```python
from build123d import *

# Parameters (mm, degrees)
SKETCH2_R           = 1.5
BOSS_EXTRUDE3_DEPTH = 3
BOSS_EXTRUDE4_DEPTH = 3
SKETCH4_R           = 1.25
CUT_EXTRUDE1_DEPTH  = 3
BOSS_EXTRUDE5_DEPTH = 3
CUT_EXTRUDE2_DEPTH  = 3
BOSS_EXTRUDE6_START = -3
SKETCH7_R           = 1.5
SKETCH7_R_2         = 1.25
BOSS_EXTRUDE6_DEPTH = 3
CUT_EXTRUDE3_DEPTH  = 10
BOSS_EXTRUDE7_DEPTH = 3


with BuildPart() as part:
    # Sketch2 → Boss-Extrude3 (new body)
    with BuildSketch(Plane.XY):
        with BuildLine():
            Line((-69.686145903, 39.746340023), (-34.686145903, 39.746340023))
            Line((-34.686145903, 39.746340023), (-34.686145903, 59.746340023))
            Line((-34.686145903, 59.746340023), (-69.686145903, 49.746340023))
            ThreePointArc((-69.686145903, 49.746340023), (-74.686145903, 44.746340023), (-69.686145903, 39.746340023))
        make_face()
        with Locations((-69.686145903, 44.746340023)):
            Circle(SKETCH2_R, mode=Mode.SUBTRACT)
    extrude(amount=BOSS_EXTRUDE3_DEPTH)

    # Sketch3 → Boss-Extrude4 (add)
    with BuildSketch(Plane.XY.offset(3)):
        with BuildLine():
            Line((-64.686145903, 39.746340023), (-59.686145903, 39.746340023))
            Line((-59.686145903, 39.746340023), (-54.686145903, 39.746340023))
            ThreePointArc((-54.686145903, 39.746340023), (-59.686145903, 34.746340023), (-64.686145903, 39.746340023))
        make_face()
    extrude(amount=-BOSS_EXTRUDE4_DEPTH)

    # Sketch4 → Cut-Extrude1 (cut)
    with BuildSketch(Plane.XY.offset(3)):
        with Locations((-59.686145903, 39.746340023)):
            Circle(SKETCH4_R)
    extrude(amount=-CUT_EXTRUDE1_DEPTH, mode=Mode.SUBTRACT)

    # Sketch5 → Boss-Extrude5 (add)
    with BuildSketch(Plane.XY.offset(3)):
        Polygon((-34.686145903, 59.746340023), (-34.686145903, 62.746340023), (-69.686145903, 49.746340023), align=None)
    extrude(amount=-BOSS_EXTRUDE5_DEPTH)

    # Sketch6 → Cut-Extrude2 (cut)
    with BuildSketch(Plane.XY.offset(3)):
        Polygon((-34.686145903, 39.746340023), (-35.686145903, 39.746340023), (-35.686145903, 63.560014977), (-33.928047703, 63.560014977), (-33.928047703, 39.746340023), align=None)
    extrude(amount=-CUT_EXTRUDE2_DEPTH, mode=Mode.SUBTRACT)

    # Sketch7 → Boss-Extrude6 (add)
    with BuildSketch(Plane.XY.offset(3).offset(BOSS_EXTRUDE6_START)):
        with Locations((-69.686145903, 44.746340023)):
            Circle(SKETCH7_R)
        with Locations((-69.686145903, 44.746340023)):
            Circle(SKETCH7_R_2, mode=Mode.SUBTRACT)
    extrude(amount=BOSS_EXTRUDE6_DEPTH)

    # Sketch8 → Cut-Extrude3 (cut)
    with BuildSketch(Plane.XY.offset(3)):
        Polygon((-69.686145903, 49.746340023), (-45.686145903, 49.746340023), (-45.686145903, 58.660625737), align=None)
    extrude(amount=-CUT_EXTRUDE3_DEPTH, mode=Mode.SUBTRACT)

    # Sketch9 → Boss-Extrude7 (add)
    with BuildSketch(Plane.XY.offset(3)):
        with BuildLine():
            Line((-59.686145903, 34.746340023), (-54.686145903, 34.746340023))
            Line((-54.686145903, 34.746340023), (-54.686145903, 39.746340023))
            ThreePointArc((-54.686145903, 39.746340023), (-56.150611997, 36.210806117), (-59.686145903, 34.746340023))
        make_face()
    extrude(amount=-BOSS_EXTRUDE7_DEPTH)


solid = part.part
```
Build history of the part. All positions in model axes, mm. A direction names the side the tool comes from. Round coordinates to 2 decimals unless told otherwise and drop trailing zeros. Write each loop counter-clockwise with the first axis right and the second up, starting at its lowest first coordinate (ties: lowest second). Pieces come first, ordered by that corner, then holes.
1) Drill centre lines: probe 1 along X at (y, z) = (53.5, 2.25); probe 2 along Y at (x, z) = (-48.5, 0.45); probe 3 along Y at (x, z) = (-55, 0.6). Where is each one in solid material? Low to high.
2) Band-saw the part on B-B, the plane y = 45.25. List the corners of the cut face in (x, z).
3) 3-axis set-ups, long thin cutter, end or side, ignore diameter. For faces 1 (the flat face through (-45, 39.746, 1)), 2 (the flat face through (-67, 39.746, 1)), 3 (the cylindrical face through (-68.53, 44.27, 1.48)), 4 (the flat face through (-45.686, 54, 2)): which of +Z, -Z, +X, -X, +Y, -Y reach the whole face in a straight line?
4) Band-saw the part on C-C, the plane y = 55.25. List the corners of the cut face in (x, z).
5) Pin check, flat tips, straight feed: pin 1 (0.9 mm diameter, centred on y = 54, z = 1.5, fed in from -X); pin 2 (4 mm diameter, centred on x = -69.69, y = 44.75, fed in from +Z); pin 3 (1.5 mm diameter, centred on x = -68, z = 2, fed in from -Y); pin 4 (0.9 mm diameter, centred on x = -63.5, z = 1.5, fed in from +Y). Stop position of each tip, or through.
6) Band-saw the part on A-A, the plane z = 1.15. List the corners of the cut face in (x, y), and give its area (3 significant figures).
7) Band-saw the part on D-D, the plane y = 41.75. List the corners of the cut face in (x, z), and give its area (3 significant figures).
8) Mould opens along Y. For faces 5 (the flat face through (-57, 34.746, 2)), 6 (the cylindrical face through (-59.109, 38.637, 1.521)), 7 (the flat face through (-35.686, 51, 2)), 8 (the flat face through (-58, 49.746, 2)) say: +Y half, -Y half, draft (parallel to the pull), parting line (faces both ways), or undercut.
Ans:
1. probe 1: x = -45.69 to -35.69
1. probe 2: y = 39.75 to 49.75
1. probe 3: y = 34.75 to 49.75
2. outline: (-74.66, 0) - (-70.83, 0) - (-70.83, 3) - (-74.66, 3) - close; (-68.54, 0) - (-35.69, 0) - (-35.69, 3) - (-68.54, 3) - close
3. face 1: +Z, -Z, +X, -Y
3. face 2: +Z, -Z, -X, -Y
3. face 3: +Z, -Z
3. face 4: +Z, -Z, -X, +Y
4. outline: (-45.69, 0) - (-35.69, 0) - (-35.69, 3) - (-45.69, 3) - close
5. pin 1: stops at x = -45.69
5. pin 2: stops at z = 3
5. pin 3: stops at y = 39.75
5. pin 4: stops at y = 49.75
6. outline: (-69.69, 39.75) - (-64.69, 39.75) arc R5 ccw to (-59.69, 34.75) - (-54.69, 34.75) - (-54.69, 39.75) - (-35.69, 39.75) - (-35.69, 62.37) - (-45.69, 58.66) - (-45.69, 49.75) - (-69.69, 49.75) arc R5 ccw to start; hole circle Ø2.5 at (-69.69, 44.75); hole circle Ø2.5 at (-59.69, 39.75)
6. area: 522 mm2
7. outline: (-73.69, 0) - (-35.69, 0) - (-35.69, 3) - (-73.69, 3) - close
7. area: 114 mm2
8. face 5: -Y half
8. face 6: undercut
8. face 7: draft
8. face 8: +Y half
